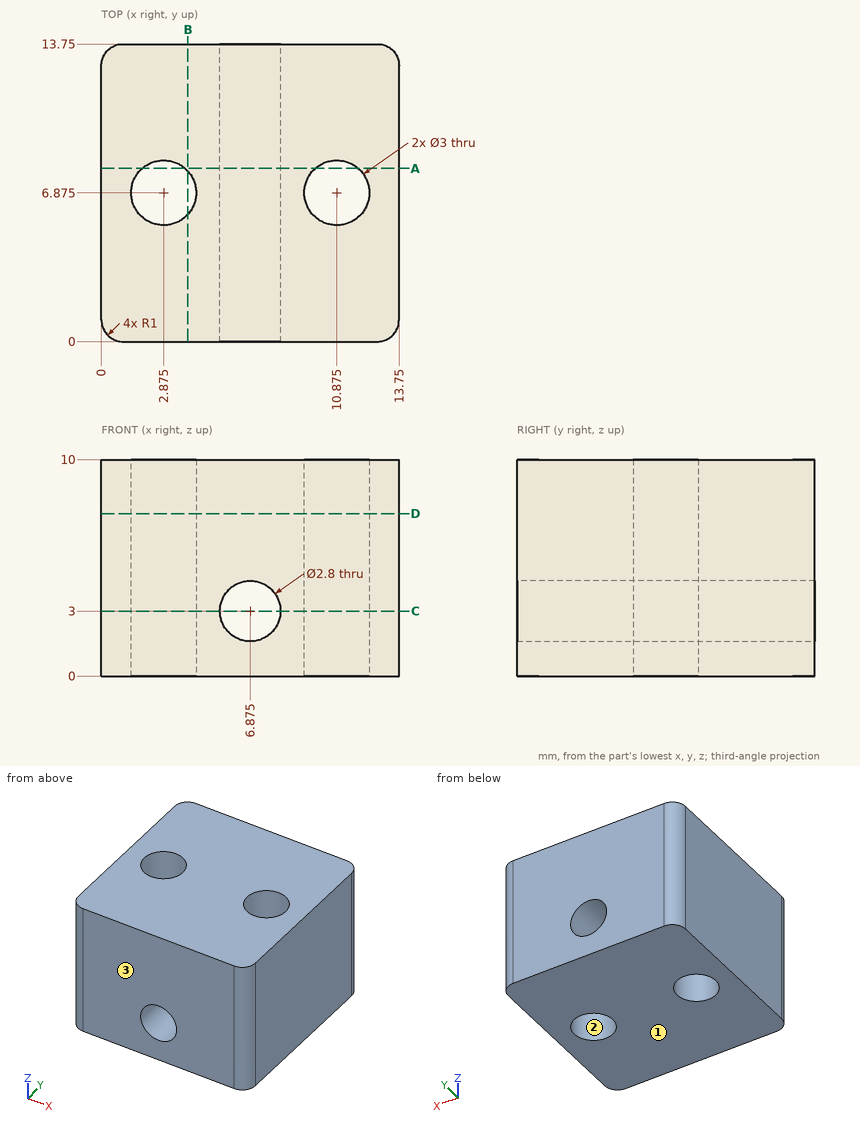
Here's the drawing with two shaded views (mm, measured from the low corner). I have some questions. Give positions to 0.01 mm unless a question says otherwise; leave off trailing zeros. Loops run counter-clockwise (first coordinate to the right, second up) from the corner with the lowest first, then second, coordinate; pieces in that order, holes last. Notation, with made-up numbers: M 72.25,82 L 122.25,82 A17 cw 122.25,113 Z; hole C 57.25,79 d8. An arc over 180 degrees is marked long. One line per item, written item: value.
(1) Will this pin go through, and if not, where does the flat tip stop? pin 1 (2 mm diameter, centred on x = 6.5, z = 3.5, fed in from -Y).
Returned:
pin 1: y = 0
(2) We'd pull the mould along Y, two halves only. Please class the marked faces 1, 2 and 3: released by +Y, released by -Y, zero draft, split by the parting line, or undercut.
Returned:
face 1: zero draft
face 2: undercut
face 3: released by -Y
(3) Suppose I cut it at D-D on z = 7.5. List the corners of the cut face in (x, y) for me (3 decimals).
Returned:
outline: M 0,1 A1 ccw 1,0 L 12.75,0 A1 ccw 13.75,1 L 13.75,12.75 A1 ccw 12.75,13.75 L 1,13.75 A1 ccw 0,12.75 Z; hole C 2.875,6.875 d3; hole C 10.875,6.875 d3
(4) Suppose I cut it at A-A on y = 8. List the corners of the cut face in (x, z) for me (3 decimals), plus the area to 3 significant figures.
Returned:
outline: M 0,0 L 1.883,0 L 1.883,10 L 0,10 Z; M 3.867,0 L 9.883,0 L 9.883,10 L 3.867,10 Z; M 11.867,0 L 13.75,0 L 13.75,10 L 11.867,10 Z; hole C 6.875,3 d2.8
area: 91.7 mm^2
(5) I need wall thicknesses on line 1 (X direction, y = 6.5, z = 8.75); line 2 (Y direction, x = 2.75, z = 2.75); line 3 (X direction, y = 6, z = 1.75). Which ranges of each line are inside material? Lowest first, please.
Returned:
line 1: 0 to 1.42, 4.33 to 9.42, 12.33 to 13.75
line 2: 0 to 5.38, 8.37 to 13.75
line 3: 0 to 1.66, 4.09 to 6.24, 7.51 to 9.66, 12.09 to 13.75
(6) Suppose I cut it at B-B on x = 4. List the corners of the cut face in (y, z) for me, plus the area to 3 significant figures.
Returned:
outline: M 0,0 L 5.88,0 L 5.88,10 L 0,10 Z; M 7.87,0 L 13.75,0 L 13.75,10 L 7.87,10 Z
area: 118 mm^2
(7) Suppose I cut it at C-C on z = 3. List the corners of the cut face in (x, y) for me (3 decimals).
Returned:
outline: M 0,1 A1 ccw 1,0 L 5.475,0 L 5.475,13.75 L 1,13.75 A1 ccw 0,12.75 Z; M 8.275,0 L 12.75,0 A1 ccw 13.75,1 L 13.75,12.75 A1 ccw 12.75,13.75 L 8.275,13.75 Z; hole C 2.875,6.875 d3; hole C 10.875,6.875 d3
